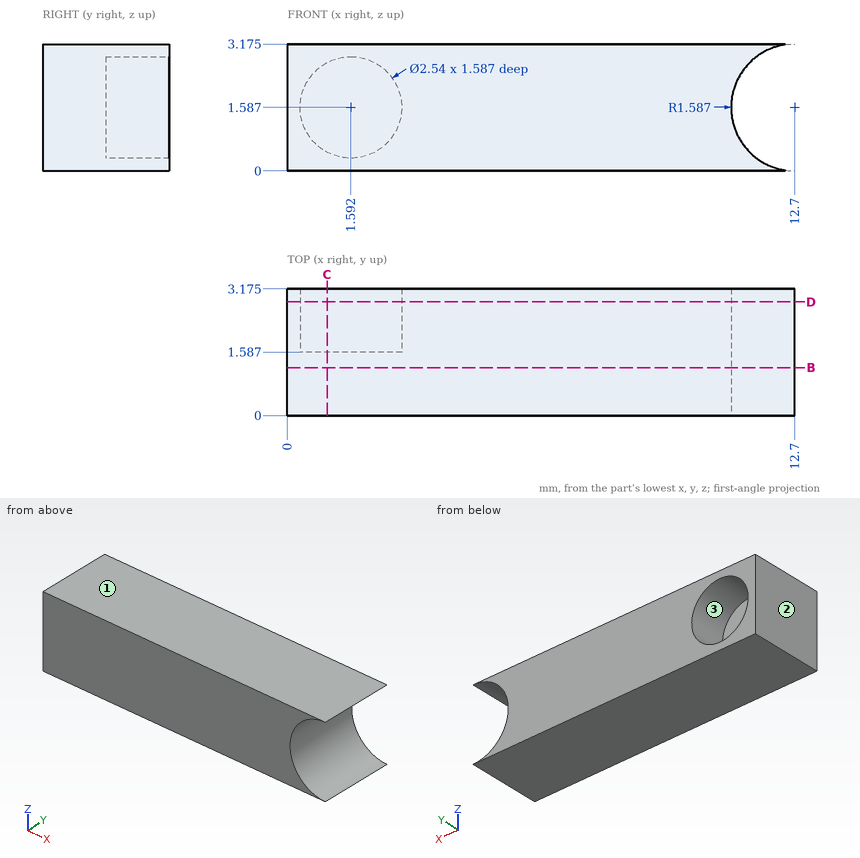
Here's the drawing with two shaded views (mm, measured from the low corner). I have some questions. Round coordinates to 2 decimals unless told otherwise and drop trailing zeros. Loops run counter-clockwise (first coordinate to the right, second up) from the corner with the lowest first, then second, coordinate; pieces in that order, holes last. Notation, with made-up numbers: M 14.25,77.5 L 29.25,77.5 A14 ccw 29.25,100.5 Z; hole C 56,-9.75 d9. An arc over 180 degrees is marked long. Put each result on its own line as item: value.
Q1. For pin 1 (1.5 mm diameter, centred on y = 2, z = 1, fed in from +X) (1 decimal), with a flat end and sliding along its axis, tell me the tip position at first contact or that it passes through.
Check result:
pin 1: x = 11.8
Q2. Imagine slicing it at C-C (x = 1). Write out the boundary of the cut face in (y, z) (1 decimal).
Check result:
outline: M 0,0 L 3.2,0 L 3.2,0.5 L 1.6,0.5 L 1.6,2.7 L 3.2,2.7 L 3.2,3.2 L 0,3.2 Z
Q3. Imagine slicing it at D-D (y = 2.85). Write out the boundary of the cut face in (x, z) (1 decimal), then the cut area to 3 significant figures.
Check result:
outline: M 0,0 L 12.7,0 A1.6 cw 12.7,3.2 L 0,3.2 Z; hole C 1.6,1.6 d2.5
area: 31.3 mm2
Q4. Imagine slicing it at B-B (y = 1.2). Write out the boundary of the cut face in (x, z) (1 decimal).
Check result:
outline: M 0,0 L 12.7,0 A1.6 cw 12.7,3.2 L 0,3.2 Z
Q5. Thinking about a two-plate mould opening in X: for the marked faces 1, 2 and 3, which applies, released by +X, released by -X, zero draft, split by the parting line, or undercut?
Check result:
face 1: zero draft
face 2: released by -X
face 3: undercut
Q6. I need wall thicknesses on probe 1 along X at (y, z) = (1.65, 2.6) (1 decimal); probe 2 along X at (y, z) = (3, 2.2) (1 decimal); probe 3 along Y at (x, z) = (1.5, 1.2). Which ranges of each line are inside material? Lowest first, please.
Check result:
probe 1: 0 to 0.8, 2.4 to 11.5
probe 2: 0 to 0.5, 2.7 to 11.2
probe 3: 0 to 1.59
